from build123d import *

# Parameters (mm, degrees)
SKETCH1_W             = 8
SKETCH1_H             = 130
BOSS_EXTRUDE1_DEPTH   = 40
SKETCH2_W             = 20.4
SKETCH2_H             = 25
CUT_EXTRUDE1_DEPTH    = 9
FILLET1_R             = 3
SKETCH3_R             = 2.2
CUT_EXTRUDE2_DEPTH    = 41
SKETCH4_W             = 56.10425639
SKETCH4_H             = 70
CUT_EXTRUDE3_DEPTH    = 7
SKETCH5_R             = 1.25
CUT_EXTRUDE4_DEPTH    = 15
CHAMFER1_SIZE         = 3
CHAMFER1_SIZE2        = 2.517298894
CHAMFER1_PART_2_SIZE  = 3
CHAMFER1_PART_2_SIZE2 = 2.517298894


with BuildPart() as part:
    # Sketch1 → Boss-Extrude1 (new body)
    with BuildSketch(Plane.XY):
        Rectangle(SKETCH1_W, SKETCH1_H)
    extrude(amount=-BOSS_EXTRUDE1_DEPTH)

    # Sketch2 → Cut-Extrude1 (cut, through all)
    with BuildSketch(Plane(origin=(4, 0, 0), x_dir=(0, 0, -1), z_dir=(1, 0, 0))):
        with Locations((20, 65)):
            Rectangle(SKETCH2_W, SKETCH2_H)
        with Locations((20, -65)):
            Rectangle(SKETCH2_W, SKETCH2_H)
    extrude(amount=-CUT_EXTRUDE1_DEPTH, mode=Mode.SUBTRACT)

    # Fillet1
    fillet1_edges = [part.edges().sort_by_distance(p)[0] for p in [
        (4, 65, -4.9),
        (-4, 65, -4.9),
        (-4, -65, -4.9),
        (4, -65, -4.9),
        (4, -65, -35.1),
        (-4, -65, -35.1),
        (-4, 65, -35.1),
        (4, 65, -35.1),
    ]]
    fillet(fillet1_edges, radius=FILLET1_R)

    # Sketch3 → Cut-Extrude2 (cut, through all)
    with BuildSketch(Plane.XY):
        with Locations((0, 60)):
            Circle(SKETCH3_R)
        with Locations((0, -60)):
            Circle(SKETCH3_R)
    extrude(amount=-CUT_EXTRUDE2_DEPTH, mode=Mode.SUBTRACT)

    # Sketch4 → Cut-Extrude3 (cut)
    with BuildSketch(Plane.XY):
        Rectangle(SKETCH4_W, SKETCH4_H)
    extrude(amount=-CUT_EXTRUDE3_DEPTH, mode=Mode.SUBTRACT)

    # Sketch5 → Cut-Extrude4 (cut)
    with BuildSketch(Plane.XY.offset(-7)):
        with Locations((0, 17.5)):
            Circle(SKETCH5_R)
        with Locations((0, -17.5)):
            Circle(SKETCH5_R)
    extrude(amount=-CUT_EXTRUDE4_DEPTH, mode=Mode.SUBTRACT)

    # Chamfer1
    chamfer1_edges = [part.edges().sort_by_distance(p)[0] for p in [
        (4, 52.5, -20),
    ]]
    chamfer1_side = [part.faces().sort_by_distance(p)[0] for p in [
        (0, 52.5, -20),
    ]]
    chamfer(chamfer1_edges, length=CHAMFER1_SIZE, length2=CHAMFER1_SIZE2, reference=chamfer1_side[0])

    # Chamfer1 part 2
    chamfer1_part_2_edges = [part.edges().sort_by_distance(p)[0] for p in [
        (4, -52.5, -20),
    ]]
    chamfer1_part_2_side = [part.faces().sort_by_distance(p)[0] for p in [
        (0, -52.5, -20),
    ]]
    chamfer(chamfer1_part_2_edges, length=CHAMFER1_PART_2_SIZE, length2=CHAMFER1_PART_2_SIZE2, reference=chamfer1_part_2_side[0])


solid = part.part
Design review of the part built by this model. Coordinates are the model's own, in mm. A direction names the side the tool comes from. Give positions to 0.01 mm unless a question says otherwise; leave off trailing zeros. Write each loop counter-clockwise with the first axis right and the second up, starting at its lowest first coordinate (ties: lowest second). Pieces come first, ordered by that corner, then holes. Notation, with made-up numbers: M 12.5,78.25 L 25.5,78.25 A35 ccw 25.5,113.25 Z; hole C 9.25,1.25 d1. An arc over 180 degrees is marked long. Answer as a JSON object with one key per item and string values. Group by question number.
1) Clearance check with flat-ended pins moving along their axes: pin 1 Ø3 at (x, y) = (0, 17.5) entering from +Z; pin 2 Ø3.5 at (x, y) = (0, 60) entering from +Z; pin 3 Ø0.8 at (x, y) = (-0.5, -17) entering from +Z; pin 4 Ø4 at (x, z) = (1.5, -27) entering from +Y. State where each tip first meets the part, or that it passes through.
2) We need section C-C (z = -19.5). Give the boundary of the cut face in (x, y).
3) We need section B-B (y = -17.5). Give the boundary of the cut face in (x, z), and give its area (4 significant figures).
4) We need section D-D (z = -33). Give the boundary of the cut face in (x, y).
5) For line 1 along Y through (x, z) = (0, -35.25); line 2 along Y through (x, z) = (0, -4.25); line 3 along Y through (x, z) = (0, -7.5), list the stretches that pass through material, from the lowest coordinate up.
6) We need section A-A (z = -5.5). Give the boundary of the cut face in (x, y), and give its area (3 significant figures).
7) Tool access review of faces 4 (the face through (-1, 52.5, -20)), 5 (the face through (-0.477, -62.148, -35.031)), 6 (the face through (0, 0, -7)), 7 (the face through (0.672, -16.446, -14.395)), 8 (the face through (-3.14, 64.1, -35.17)): name each direction out of +Z, -Z, +X, -X, +Y, -Y from which nothing blocks a thin tool from reaching the whole face with its end or side.
8) Mouldability with a two-part tool opening along Z and no side actions: class faces 1 (the face through (0, 1, -40)), 2 (the face through (3.1, 64.14, -4.97)), 3 (the face through (-1, -52.5, -20)) as released by +Z, released by -Z, zero draft, split by the parting line, or undercut.
Answer key:
{
 "1": {"pin 1": "stops at z = -7", "pin 2": "passes through", "pin 3": "stops at z = -22", "pin 4": "stops at y = 52.5"},
 "2": {"outline": "M -4,-52.5 L 1,-52.5 L 4,-49.98 L 4,49.98 L 1,52.5 L -4,52.5 Z; hole C 0,-17.5 d2.5; hole C 0,17.5 d2.5"},
 "3": {"outline": "M -4,-40 L 4,-40 L 4,-7 L 1.25,-7 L 1.25,-22 L -1.25,-22 L -1.25,-7 L -4,-7 Z", "area": "226.5 mm²"},
 "4": {"outline": "M -4,-62 A3 ccw -1,-65 L 1,-65 A3 ccw 4,-62 L 4,62 A3 ccw 1,65 L -1,65 A3 ccw -4,62 Z; hole C 0,-60 d4.4; hole C 0,60 d4.4"},
 "5": {"line 1": "y = -65 to -62.2, -57.8 to 57.8, 62.2 to 65", "line 2": "y = -65 to -62.2, -57.8 to -35, 35 to 57.8, 62.2 to 65", "line 3": "y = -65 to -62.2, -57.8 to -18.75, -16.25 to 16.25, 18.75 to 57.8, 62.2 to 65"},
 "6": {"outline": "M -4,-62 A3 ccw -1,-65 L 1,-65 A3 ccw 4,-62 L 4,-35 L -4,-35 Z; M -4,35 L 4,35 L 4,62 A3 ccw 1,65 L -1,65 A3 ccw -4,62 Z; hole C 0,-60 d4.4; hole C 0,60 d4.4", "area": "442 mm²"},
 "7": {"face 4": "+X, -X, +Y", "face 5": "+Z, -Z", "face 6": "+Z, +X, -X", "face 7": "+Z", "face 8": "+Z, -Z, -X, +Y"},
 "8": {"face 1": "released by -Z", "face 2": "zero draft", "face 3": "undercut"}
}
